CAD build for the part. Positions are in the model's coordinates, mm. A direction names the side the tool comes from. Give positions to 0.01 mm unless a question says otherwise; leave off trailing zeros. Write each loop counter-clockwise with the first axis right and the second up, starting at its lowest first coordinate (ties: lowest second). Pieces come first, ordered by that corner, then holes. Notation, with made-up numbers: (-21.5, 83) -> (17.5, 83) arc R10 cw to (17.5, 102) -> close; hole circle Ø2 at (37, 18). An arc over 180 degrees is marked (long way). Answer as a JSON object with one key per item and string values.
```python
from build123d import *

# Parameters (mm, degrees)
EXTRUDE_START   = 0.1
SKETCH_2_W      = 6
SKETCH_2_H      = 6
EXTRUDE_1_DEPTH = 3
CHAMFER_1_SIZE  = 1.18


with BuildPart() as part:
    # Эскиз1 → Повернуть1 (revolve)
    with BuildSketch(Plane.XY, mode=Mode.PRIVATE) as revolve_1_sk:
        with BuildLine():
            Line((25, 0), (25, 2.95))
            Line((25, 2.95), (7.1, 2.95))
            Line((7.1, 2.95), (7.1, 3))
            Line((7.1, 3), (0, 3))
            Line((0, 3), (0, 7))
            Line((0, 7), (-1.124355653, 7))
            ThreePointArc((-1.124355653, 7), (-2.522961568, 3.623466631), (-3, 0))
            Line((-3, 0), (25, 0))
        make_face()
    revolve(revolve_1_sk.sketch.rotate(Axis((-121.430503085, 0, 0), (1, 0, 0)), 90), axis=Axis((-121.430503085, 0, 0), (1, 0, 0)))

    # Эскиз2 → Бобышка-Вытянуть1 (add)
    with BuildSketch(Plane(origin=(0, 0, 0), x_dir=(0, 0, -1), z_dir=(1, 0, 0)).offset(EXTRUDE_START)):
        Rectangle(SKETCH_2_W, SKETCH_2_H)
    extrude(amount=EXTRUDE_1_DEPTH)

    # Фаска1
    chamfer_1_edges = [part.edges().sort_by_distance(p)[0] for p in [
        (25, 0, -2.95),
    ]]
    chamfer(chamfer_1_edges, length=CHAMFER_1_SIZE)


solid = part.part
```
1) Pin check, flat tips, straight feed: pin 1 (0.9 mm diameter, centred on y = 2, z = -1, fed in from -X); pin 2 (6 mm diameter, centred on x = 0, y = -3, fed in from +Z); pin 3 (1.5 mm diameter, centred on y = 1, z = 1.5, fed in from -X); pin 4 (1.5 mm diameter, centred on x = 14.5, y = 1, fed in from +Z). Stop position of each tip, or through.
Model answer:
{"pin 1": "stops at x = -2.89", "pin 2": "stops at z = 7", "pin 3": "stops at x = -2.96", "pin 4": "stops at z = 2.94"}
2) Slice it at A-A (x = 17). List the corners of the cut face in (y, z), then the cut area to 3 significant figures.
Model answer:
{"outline": "circle Ø5.9 at (0, 0)", "area": "27.3 mm2"}
3) Wall check: probe 1 along X at (y, z) = (-2.5, -4.5); probe 2 along Y at (x, z) = (19.25, -1.5); probe 3 along Y at (x, z) = (15.25, 2). Give the ranges that are in metal, low to high.
Model answer:
{"probe 1": "x = -2.02 to 0", "probe 2": "y = -2.54 to 2.54", "probe 3": "y = -2.17 to 2.17"}
4) Slice it at D-D (x = 3.75). List the corners of the cut face in (y, z).
Model answer:
{"outline": "circle Ø6 at (0, 0)"}
5) Slice it at B-B (y = 3.75). List the corners of the cut face in (x, z).
Model answer:
{"outline": "(-1.12, -5.91) -> (0, -5.91) -> (0, 5.91) -> (-1.12, 5.91) arc R13.49 ccw to start"}
6) Slice it at C-C (z = -4.5). List the corners of the cut face in (x, y), then the cut area to 3 significant figures.
Model answer:
{"outline": "(-1.12, -5.36) -> (0, -5.36) -> (0, 5.36) -> (-1.12, 5.36) arc R13.26 ccw to start", "area": "20.2 mm2"}
7) 3-axis set-ups, long thin cutter, end or side, ignore diameter. For faces 1 (the flat face through (3.1, 2.3, 2.4)), 2 (the flat face through (3.1, -2.3, 2.4)), 3 (the flat face through (2, 0, 3)), 4 (the cylindrical face through (5.07, -0.9, 2.86)): which of +Z, -Z, +X, -X, +Y, -Y reach the whole face in a straight line?
Model answer:
{"face 1": "+Z, +X, +Y", "face 2": "+Z, +X, -Y", "face 3": "+Z, +X, +Y, -Y", "face 4": "+X"}
